The model under review builds one solid part; all positions refer to its coordinate system, in mm. A direction names the side the tool comes from. Round coordinates to 2 decimals unless told otherwise and drop trailing zeros. Loops run counter-clockwise (first coordinate to the right, second up) from the corner with the lowest first, then second, coordinate; pieces in that order, holes last. Notation, with made-up numbers: M -15,66 L -8,66 A26 ccw -8,103 Z; hole C -27.75,22 d9. An arc over 180 degrees is marked long. Return JSON: item names as keys, results as strings. Group by question number.
Q1. Consider section A-A (x = 0). State the section outline as (y, z) points.
Q2. Consider section B-B (y = -6.5). State the section outline as (x, z) points.
Q3. For faces 4 (the face through (25, -40, 7)), 5 (the face through (0, -40, 7)), list the 3-axis set-ups (+Z, -Z, +X, -X, +Y, -Y) from which the entire face can be reached by the end or side of a thin tool; tool diameter is ignored.
Q4. Consider section D-D (y = -18). State the section outline as (x, z) points.
Q5. Clearance check with flat-ended pins moving along their axes: pin 1 Ø4 at (x, z) = (-5.5, 3) entering from -Y; pin 2 Ø3 at (y, z) = (-25, 3.5) entering from +X; pin 3 Ø1.5 at (x, z) = (-8, 12.5) entering from +Y. State where each tip first meets the part, or that it passes through.
Q6. To check wall thickness, follow line 1 along X through (y, z) = (-5, 4.5); line 2 along Y through (x, z) = (-8, 5); line 3 along X through (y, z) = (-15, 2). State the ranges of each line that lie inside material, in increasing order.
Q7. Consider section C-C (z = 3.25). State the section outline as (x, y) points, and give its area (3 significant figures).
Q8. Draft analysis for pull direction X (two halves, no side actions). For faces 1 (the face through (19.666, -15.27, 7.395)), 2 (the face through (18, -45, 7)), 3 (the face through (-11, -43, 7)), state which applies: pulls with the +X half, pulls with the -X half, needs draft (parallel to the pull), parting line crosses it, or undercut.
Autodesk Inventor part; units mm, degrees
ref_plane "YZ Plane" through (0, 0, 0) normal (1, 0, 0) x (0, 1, 0)
ref_plane "XZ Plane" through (0, 0, 0) normal (0, 1, 0) x (-1, 0, 0)
ref_plane "XY Plane" through (0, 0, 0) normal (0, 0, 1) x (1, 0, 0)
sketch "草图1" plane through (0, 0, 0) normal (0, 0, 1) x (1, 0, 0)
  line L0 (0, 7.9673) -> (0, -10.1658)
  circle A0 centre (0, 0) radius 9
  line L1 (-14.4802, 3.9145) -> (-25, -35)
  line L2 (14.4802, 3.9145) -> (25, -35)
  line L3 (-25, -35) -> (-25, -45)
  line L4 (-25, -45) -> (-11, -45)
  line L5 (-11, -45) -> (-11, -40)
  line L6 (-11, -40) -> (11, -40)
  line L7 (11, -40) -> (11, -45)
  line L8 (25, -45) -> (11, -45)
  line L9 (25, -35) -> (25, -45)
  arc A1 (14.4802, 3.9145) -> (-14.4802, 3.9145) centre (0, 0) ccw
  dimension "d1" = 18
  dimension "d2" = 22
  dimension "d3" = 50
  dimension "d4" = 5
  dimension "d5" = 10
  dimension "d6" = 45
  dimension "d7" = 15
extrude "拉伸1" add sketch "草图1" along normal blind 15
Values:
{
 "1": {"outline": "M -40,0 L -9,0 L -9,15 L -40,15 Z; M 9,0 L 15,0 L 15,15 L 9,15 Z"},
 "2": {"outline": "M -17.3,0 L -6.22,0 L -6.22,15 L -17.3,15 Z; M 6.22,0 L 17.3,0 L 17.3,15 L 6.22,15 Z"},
 "3": {"face 4": "+Z, -Z, +X, +Y, -Y", "face 5": "+Z, -Z, -Y"},
 "4": {"outline": "M -20.4,0 L 20.4,0 L 20.4,15 L -20.4,15 Z"},
 "5": {"pin 1": "stops at y = -40", "pin 2": "stops at x = 22.7", "pin 3": "stops at y = 13.13"},
 "6": {"line 1": "x = -16.89 to -7.48, 7.48 to 16.89", "line 2": "y = -40 to -4.12, 4.12 to 12.69", "line 3": "x = -19.59 to 19.59"},
 "7": {"outline": "M -25,-45 L -11,-45 L -11,-40 L 11,-40 L 11,-45 L 25,-45 L 25,-35 L 14.48,3.91 A15 ccw -14.48,3.91 L -25,-35 Z; hole C 0,0 d18", "area": "1,910 mm2"},
 "8": {"face 1": "pulls with the +X half", "face 2": "needs draft", "face 3": "undercut"}
}
